The figure shows three views and two pictorial views of one solid part (mm, origin at its lowest corner). Answer the questions. A direction names the side the tool comes from. Coordinates: 2 decimals unless noted, no trailing zeros. Write each loop counter-clockwise with the first axis right and the second up, starting at its lowest first coordinate (ties: lowest second). Pieces come first, ordered by that corner, then holes.
Item 1: Straight lines are drawn through the part: probe 1 along Z at (x, y) = (3, 1.65); probe 2 along X at (y, z) = (1.1, 2.25) (1 decimal); probe 3 along X at (y, z) = (1.2, 4.5). For each, find the intervals that lie inside material, in ascending order.
Item 2: Section B-B (y = 1.8) is taken. Give the vertices of the cut face in (x, z).
Item 3: A tool of negligible diameter and unlimited length cuts with its end or side. For the marked faces 1 and 2, from which of +Z, -Z, +X, -X, +Y, -Y can it reach the whole face along a straight path? Write none if from no direction.
Item 4: Section A-A (x = 2.75) is taken. Give the vertices of the cut face in (y, z).
Item 5: Section C-C (z = 4) is taken. Give the vertices of the cut face in (x, y).
Item 6: Determine the mould class of the marked faces 3, 4, 5 and 6 for opening direction Z: released by +Z, released by -Z, zero draft, split by the parting line, or undercut.
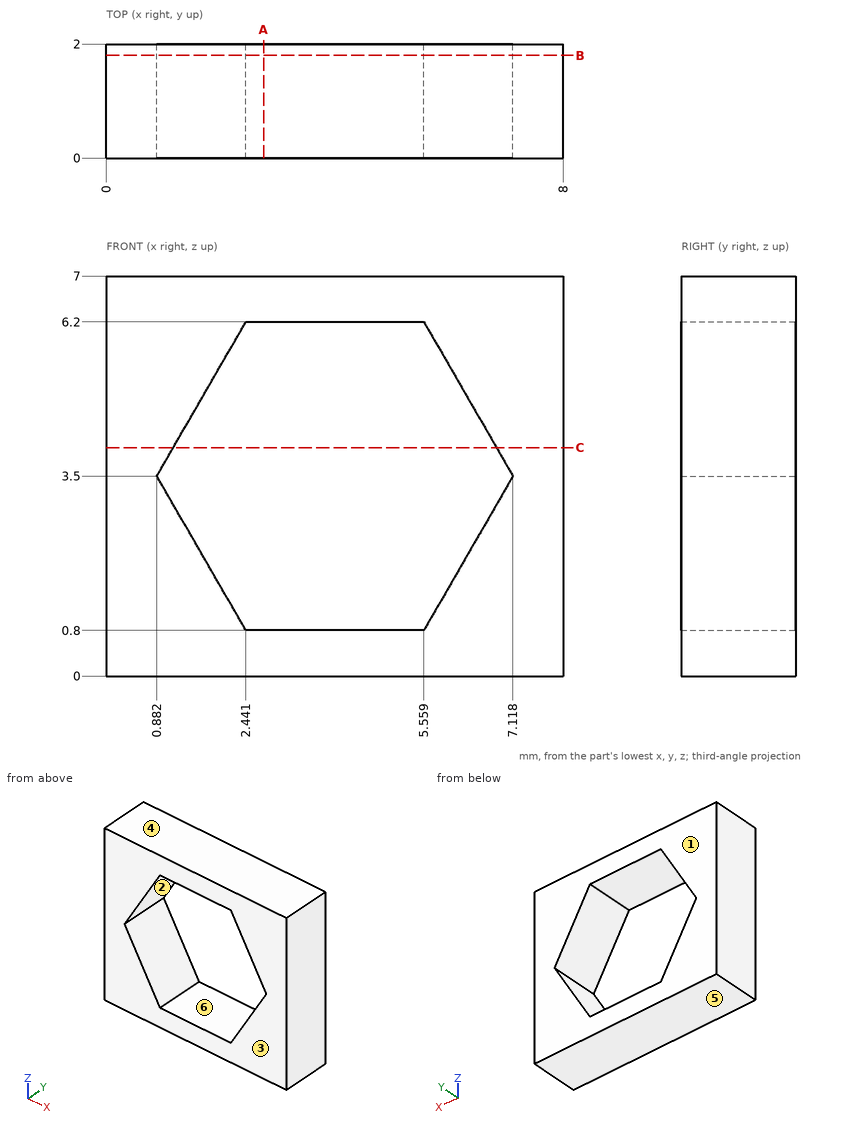
Established:
1. probe 1: z = 0 to 0.8, 6.2 to 7
1. probe 2: x = 0 to 1.6, 6.4 to 8
1. probe 3: x = 0 to 1.46, 6.54 to 8
2. outline: (0, 0) - (8, 0) - (8, 7) - (0, 7) - close; hole (0.88, 3.5) - (2.44, 0.8) - (5.56, 0.8) - (7.12, 3.5) - (5.56, 6.2) - (2.44, 6.2) - close
3. face 1: +Z, -Z, +X, -X, +Y
3. face 2: +Y, -Y
4. outline: (0, 0) - (2, 0) - (2, 0.8) - (0, 0.8) - close; (0, 6.2) - (2, 6.2) - (2, 7) - (0, 7) - close
5. outline: (0, 0) - (1.17, 0) - (1.17, 2) - (0, 2) - close; (6.83, 0) - (8, 0) - (8, 2) - (6.83, 2) - close
6. face 3: zero draft
6. face 4: released by +Z
6. face 5: released by -Z
6. face 6: undercut
